```python
from build123d import *

# Parameters (mm, degrees)
F1_DEPTH = 2.54
F2_R     = 0.849257
F2_R_2   = 1.467639
F2_R_3   = 1.986785
F2_R_4   = 1.103769
F2_R_5   = 1.035394
F2_R_6   = 1.385658
F3_DEPTH = 0.254


with BuildPart() as f1:
    # F0 (on Top) → F1 (new body)
    with BuildSketch(Plane.XY):
        with BuildLine():
            Line((-1.269909, 0.074241), (-1.269909, -6.349547))
            Line((-1.269909, -6.349547), (1.269909, -6.349547))
            Line((1.269909, -6.349547), (1.269909, 0.111635))
            ThreePointArc((1.269909, 0.111635), (0.001368, 2e-05), (-1.269909, 0.074241))
        make_face()
        with BuildLine():
            Line((-1.269909, 6.349547), (-1.269909, 0.074241))
            ThreePointArc((-1.269909, 0.074241), (0.001368, 2e-05), (1.269909, 0.111635))
            Line((1.269909, 0.111635), (1.269909, 6.349547))
            Line((1.269909, 6.349547), (-1.269909, 6.349547))
        make_face()
        with BuildLine():
            Line((-8.52301, 6.349547), (-1.269909, 6.349547))
            Line((-1.269909, 6.349547), (1.269909, 6.349547))
            Line((1.269909, 6.349547), (8.268841, 6.349547))
            ThreePointArc((8.268841, 6.349547), (-0.127084, 17.449755), (-8.52301, 6.349547))
        make_face()
    extrude(amount=F1_DEPTH)

    # F2 (on face) → F3 (join)
    with BuildSketch(Plane.XY.offset(2.54)):
        with Locations((-3.528252, 12.866852)):
            Circle(F2_R)
        with Locations((3.777331, 8.522992)):
            Circle(F2_R_2)
        with Locations((1.901574, 13.656645)):
            Circle(F2_R_3)
        with Locations((-4.318044, 8.819164)):
            Circle(F2_R_4)
        with Locations((-0.127084, 8.724415)):
            Circle(F2_R_5)
        with Locations((-1.455046, 15.433677)):
            Circle(F2_R_6)
    extrude(amount=F3_DEPTH)

    # F4: F1 across plane


with BuildPart() as f1_1:
    add(f1.part)
    add(f1.part.mirror(Plane.XY))


solid = f1_1.part
```
CAD build for the part. Positions are in the model's coordinates, mm. A direction names the side the tool comes from. Give positions to 0.01 mm unless a question says otherwise; leave off trailing zeros. Write each loop counter-clockwise with the first axis right and the second up, starting at its lowest first coordinate (ties: lowest second). Pieces come first, ordered by that corner, then holes. Notation, with made-up numbers: M -20.5,20 L -12.5,20 A31 cw -12.5,59 Z; hole C 53,-28 d6. An arc over 180 degrees is marked long. Return JSON: item names as keys, results as strings. Group by question number.
(1) Flat gauge pins, fed straight in: pin 1 Ø1.5 at (x, z) = (4.5, 0) entering from -Y; pin 2 Ø6 at (x, y) = (1.5, -2) entering from -Z; pin 3 Ø1.5 at (y, z) = (2.5, -1) entering from +X; pin 4 Ø3 at (y, z) = (9.5, 0) entering from -X. Where does each tip first touch, or does it go through?
(2) Band-saw the part on B-B (z = -1.85). Give the cut face in (x, y).
(3) 3-axis set-ups, long thin cutter, end or side, ignore diameter. For faces 1 (the face through (0, 10, 2.54)), 2 (the face through (-5, 6.35, 0)), 3 (the face through (0, 10, -2.54)), 4 (the face through (0.098, 17.447, 0.036)), 5 (the face through (5, 6.35, 0)): which of +Z, -Z, +X, -X, +Y, -Y reach the whole face in a straight line?
(4) Band-saw the part on D-D (x = -3.75). Give the cut face in (y, z).
(5) Band-saw the part on C-C (y = 0). Give the cut face in (x, z), and give its area (3 significant figures).
(6) Drill centre lines: L1, parallel to Z at x = -6.25, y = 11.25; L2, parallel to X at y = -2.5, z = 0.9; L3, parallel to X at y = 8.5, z = 1.6. Where is each one in solid material? Low to high. Write a range as [from, to].
(7) Band-saw the part on A-A (x = 5). Give the cut face in (y, z).
Entries:
{
 "1": {"pin 1": "stops at y = 6.35", "pin 2": "stops at z = -2.54", "pin 3": "stops at x = 1.27", "pin 4": "stops at x = -8.85"},
 "2": {"outline": "M -8.52,6.35 L -1.27,6.35 L -1.27,-6.35 L 1.27,-6.35 L 1.27,6.35 L 8.27,6.35 A8.73 ccw long Z"},
 "3": {"face 1": "+Z", "face 2": "+Z, -Z, -X, -Y", "face 3": "-Z", "face 4": "+Z, -Z", "face 5": "+Z, -Z, +X, -Y"},
 "4": {"outline": "M 6.35,-2.54 L 7.87,-2.54 L 7.87,-2.79 L 9.77,-2.79 L 9.77,-2.54 L 12.05,-2.54 L 12.05,-2.79 L 13.69,-2.79 L 13.69,-2.54 L 16.66,-2.54 L 16.66,2.54 L 13.69,2.54 L 13.69,2.79 L 12.05,2.79 L 12.05,2.54 L 9.77,2.54 L 9.77,2.79 L 7.87,2.79 L 7.87,2.54 L 6.35,2.54 Z"},
 "5": {"outline": "M -1.27,-2.54 L 1.27,-2.54 L 1.27,2.54 L -1.27,2.54 Z", "area": "12.9 mm^2"},
 "6": {"L1": "z = [-2.54, 2.54]", "L2": "x = [-1.27, 1.27]", "L3": "x = [-8.85, 8.6]"},
 "7": {"outline": "M 6.35,-2.54 L 7.71,-2.54 L 7.71,-2.79 L 9.33,-2.79 L 9.33,-2.54 L 15.78,-2.54 L 15.78,2.54 L 9.33,2.54 L 9.33,2.79 L 7.71,2.79 L 7.71,2.54 L 6.35,2.54 Z"}
}
